The listing builds one solid part. Answer for the finished solid, in the listing's coordinates (mm). A direction names the side the tool comes from. Give positions to 0.01 mm unless a question says otherwise; leave off trailing zeros. Write each loop counter-clockwise with the first axis right and the second up, starting at its lowest first coordinate (ties: lowest second). Pieces come first, ordered by that corner, then holes. Notation, with made-up numbers: (-39, 67) - (-7, 67) arc R35 ccw to (-7, 103) - close; hole circle Ø9 at (-26.75, -10.75). An arc over 180 degrees is marked (long way). Answer in a Markdown table with one row per item. Add a question column.
from build123d import *

# Parameters (mm, degrees)
SKETCH1_W           = 90
SKETCH1_H           = 70
BOSS_EXTRUDE1_DEPTH = 1.6
SKETCH2_R           = 1.5
CUT_EXTRUDE1_DEPTH  = 1.6
SKETCH3_W           = 5
SKETCH3_H           = 39
BOSS_EXTRUDE2_DEPTH = 19
SKETCH4_W           = 26
SKETCH4_H           = 50
SKETCH4_W_2         = 13
SKETCH4_H_2         = 17
BOSS_EXTRUDE3_DEPTH = 15.5
SKETCH5_W           = 9
SKETCH5_H           = 14
BOSS_EXTRUDE4_DEPTH = 13.6
SKETCH6_R           = 2.7
CUT_EXTRUDE2_DEPTH  = 8
FILLET1_START       = -28.6
FILLET1_DEPTH       = 10.6
SKETCH7_W           = 12
SKETCH7_H           = 4.5
BOSS_EXTRUDE5_DEPTH = 9


with BuildPart() as part:
    # Sketch1 → Boss-Extrude1 (new body)
    with BuildSketch(Plane(origin=(0, 0, 0), x_dir=(1, 0, 0), z_dir=(0, 1, 0))):
        Rectangle(SKETCH1_W, SKETCH1_H)
    extrude(amount=BOSS_EXTRUDE1_DEPTH)

    # Sketch2 → Cut-Extrude1 (cut)
    with BuildSketch(Plane(origin=(0, 1.6, 0), x_dir=(1, 0, 0), z_dir=(0, 1, 0))):
        with Locations(Location((-41.5, 32.5, 0), (0, 0, 270))):
            Circle(SKETCH2_R)
        with Locations(Location((41.5, 32.5, 0), (0, 0, 270))):
            Circle(SKETCH2_R)
        with Locations(Location((41.5, -32.5, 0), (0, 0, 270))):
            Circle(SKETCH2_R)
        with Locations(Location((-41.5, -32.5, 0), (0, 0, 270))):
            Circle(SKETCH2_R)
    extrude(amount=-CUT_EXTRUDE1_DEPTH, mode=Mode.SUBTRACT)

    # Sketch3 → Boss-Extrude2 (add)
    with BuildSketch(Plane(origin=(0, 1.6, 0), x_dir=(1, 0, 0), z_dir=(0, 1, 0))):
        with Locations((-24.5, -5)):
            Rectangle(SKETCH3_W, SKETCH3_H)
    extrude(amount=BOSS_EXTRUDE2_DEPTH)

    # Sketch4 → Boss-Extrude3 (add)
    with BuildSketch(Plane(origin=(0, 1.6, 0), x_dir=(1, 0, 0), z_dir=(0, 1, 0))):
        with Locations((19, 6)):
            Rectangle(SKETCH4_W, SKETCH4_H)
        with Locations((-2.5, 5.5)):
            Rectangle(SKETCH4_W_2, SKETCH4_H_2)
    extrude(amount=BOSS_EXTRUDE3_DEPTH)

    # Sketch5 → Boss-Extrude4 (add)
    with BuildSketch(Plane(origin=(0, 1.6, 0), x_dir=(1, 0, 0), z_dir=(0, 1, 0))):
        with Locations((-32.5, 25)):
            Rectangle(SKETCH5_W, SKETCH5_H)
    extrude(amount=BOSS_EXTRUDE4_DEPTH)

    # Sketch6 → Cut-Extrude2 (cut)
    with BuildSketch(Plane(origin=(0, 0, -32), x_dir=(-1, 0, 0), z_dir=(0, 0, -1))):
        with Locations((32.5, 10.7)):
            Circle(SKETCH6_R)
    extrude(amount=-CUT_EXTRUDE2_DEPTH, mode=Mode.SUBTRACT)

    # Fillet1: read off the stored shape, not the designer's step
    # Fillet1 outline → Fillet1 (cut)
    with BuildSketch(Plane.XY.offset(FILLET1_START)):
        with BuildLine():
            Line((-28, 15.2), (-32.5, 15.2))
            ThreePointArc((-32.5, 15.2), (-29.318019485, 13.881980515), (-28, 10.7))
            Line((-28, 10.7), (-28, 15.2))
        make_face()
        with BuildLine():
            ThreePointArc((-37, 10.7), (-35.681980515, 13.881980515), (-32.5, 15.2))
            Line((-32.5, 15.2), (-37, 15.2))
            Line((-37, 15.2), (-37, 10.7))
        make_face()
    extrude(amount=FILLET1_DEPTH, mode=Mode.SUBTRACT)

    # Sketch7 → Boss-Extrude5 (add)
    with BuildSketch(Plane(origin=(0, 1.6, 0), x_dir=(1, 0, 0), z_dir=(0, 1, 0))):
        with Locations((-9, 30.45)):
            Rectangle(SKETCH7_W, SKETCH7_H)
    extrude(amount=BOSS_EXTRUDE5_DEPTH)


solid = part.part
1. A tool of negligible diameter and unlimited length cuts with its end or side. For faces 4 (the face through (-33, 7, -32)), 5 (the face through (-22, 11, 5)), 6 (the face through (-9, 9, -5)), 7 (the face through (19, 9, -31)), from which of +Z, -Z, +X, -X, +Y, -Y can it reach the whole face along a straight path? Write none if from no direction.
2. The mould has two halves that part along Y. Classify faces 1 (the face through (-32, 11, -24)), 2 (the face through (-1, 0, 0)), 3 (the face through (-25, 11, 24.5)): +Y half, -Y half, draft (parallel to the pull), parting line (faces both ways), or undercut.
3. Section D-D (z = -15.5) is taken. Give the vertices of the cut face in (x, y).
4. Section C-C (x = -41.5) is taken. Give the vertices of the cut face in (y, z), and give its area (3 significant figures).
5. Section B-B (y = 4.5) is taken. Give the vertices of the cut face in (x, z).
6. Straight lines are drawn through the part: L1, parallel to X at y = 1.15, z = -32.5; L2, parallel to X at y = 5.25, z = -11; L3, parallel to X at y = 5, z = 18.5. For each, find the intervals that lie inside material, in ascending order. Write a range as [from, to].
7. Given pin 1 Ø8 at (x, z) = (25.5, 7.5) entering from -Y; pin 2 Ø1.5 at (x, z) = (3, 9) entering from +Y; pin 3 Ø1.4 at (y, z) = (5.5, -29.5) entering from -X; pin 4 Ø4 at (y, z) = (9.5, -25.5) entering from +X, each flat-ended and moving along its own axis, determine where each tip first touches the part or whether it passes through.
8. Section A-A (z = 32.5) is taken. Give the vertices of the cut face in (x, y).
Geometry check:
| question | item | result |
|---|---|---|
| 1 | face 4 | -Z, -X, +Y |
| 1 | face 5 | +Z, -Z, +Y |
| 1 | face 6 | +Z, +Y |
| 1 | face 7 | -Z, +X, +Y |
| 2 | face 1 | undercut |
| 2 | face 2 | -Y half |
| 2 | face 3 | draft |
| 3 | outline | (-45, 0) - (45, 0) - (45, 1.6) - (32, 1.6) - (32, 17.1) - (6, 17.1) - (6, 1.6) - (-45, 1.6) - close |
| 4 | outline | (0, -35) - (1.6, -35) - (1.6, -34) - (0, -34) - close; (0, -31) - (1.6, -31) - (1.6, 31) - (0, 31) - close; (0, 34) - (1.6, 34) - (1.6, 35) - (0, 35) - close |
| 4 | area | 102 mm² |
| 5 | outline | (-37, -32) - (-28, -32) - (-28, -18) - (-37, -18) - close; (-27, -14.5) - (-22, -14.5) - (-22, 24.5) - (-27, 24.5) - close; (-15, -32.7) - (-3, -32.7) - (-3, -28.2) - (-15, -28.2) - close; (-9, -14) - (4, -14) - (4, 3) - (-9, 3) - close; (6, -31) - (32, -31) - (32, 19) - (6, 19) - close |
| 6 | L1 | [-45, -43], [-40, 40], [43, 45] |
| 6 | L2 | [-27, -22], [-9, 4], [6, 32] |
| 6 | L3 | [-27, -22], [6, 32] |
| 7 | pin 1 | y = 0 |
| 7 | pin 2 | y = 1.6 |
| 7 | pin 3 | x = -37 |
| 7 | pin 4 | x = 32 |
| 8 | outline | (-45, 0) - (-43, 0) - (-43, 1.6) - (-45, 1.6) - close; (-40, 0) - (40, 0) - (40, 1.6) - (-40, 1.6) - close; (43, 0) - (45, 0) - (45, 1.6) - (43, 1.6) - close |
